Build history of the part. All positions in model axes, mm. A direction names the side the tool comes from. Coordinates: 2 decimals unless noted, no trailing zeros. Order: outer loops, then holes, each group sorted by start corner. A loop starts at its lowest first (then second) coordinate and runs counter-clockwise, first axis right, second up. Notation, with made-up numbers: M 27,80 L 77,80 A31 cw 77,111 Z; hole C 66.5,-18 d2. An arc over 180 degrees is marked long. Write item = value, one per line. Start each with the question number.
Q1. Pull direction X, two halves, no side cores. Call faces 1 (the face through (0, -7, 0)), 2 (the face through (18.417, -4.984, 14.383)), 3 (the face through (-3, -22, 20)): released by +X, released by -X, zero draft, split by the parting line, or undercut.
Q2. Band-saw the part on D-D on x = -4. Write the cut outline in (y, z), plus the area to 3 significant figures.
Q3. Drill centre lines: probe 1 along X at (y, z) = (-5.75, 6); probe 2 along X at (y, z) = (-13, 37.5); probe 3 along Y at (x, z) = (17, 22.5). Where is each one in solid material? Low to high.
Q4. Band-saw the part on C-C on y = -15. Write the cut outline in (x, z), plus the area to 3 significant figures.
Q5. Band-saw the part on A-A on x = -20. Write the cut outline in (y, z) (3 decimals), plus the area to 3 significant figures.
Q6. Pin check, flat tips, straight feed: P1, Ø5, axis at x = 1.5, y = -7.5, coming from the +Z side; P2, Ø7, axis at x = -20, z = 6, coming from the +Y side; P3, Ø4, axis at x = -12.5, z = 28.5, coming from the -Y side; P4, Ø17, axis at y = -5.34, z = 22.5, coming from the -X side. Stop position of each tip, or through.
Q7. Band-saw the part on B-B on z = 6. State how many separate pieces and enclosed holes the cut face has, plus the area to 3 significant figures.
Q8. 3-axis set-ups, long thin cutter, end or side, ignore diameter. For faces 4 (the face through (22.948, -5.055, 16.006)), 5 (the face through (24.46, 6.69, 5.41)), 6 (the face through (15.952, -12, 29)): which of +Z, -Z, +X, -X, +Y, -Y reach the whole face in a straight line?
```python
from build123d import *

# Parameters (mm, degrees)
BOSS_EXTRUDE1_DEPTH = 40
SKETCH2_R           = 2.6
BOSS_EXTRUDE2_DEPTH = 9
SKETCH3_R           = 4.5
CUT_EXTRUDE1_DEPTH  = 5
SKETCH4_R           = 2.6
CUT_EXTRUDE2_DEPTH  = 59.309518948
CHAMFER1_SIZE       = 3
SKETCH5_R           = 6.5
CUT_EXTRUDE3_DEPTH  = 55
SKETCH6_R           = 8.125
CUT_EXTRUDE4_DEPTH  = 5
CUT_EXTRUDE5_START  = -5
SKETCH7_R           = 8.125
CUT_EXTRUDE5_DEPTH  = 5
SKETCH8_R           = 8.125
CUT_EXTRUDE6_DEPTH  = 5
SKETCH9_R           = 4.5
CUT_EXTRUDE7_DEPTH  = 4
CHAMFER2_SIZE       = 3
SKETCH10_W          = 6
SKETCH10_H          = 40
BOSS_EXTRUDE3_DEPTH = 2
CUT_EXTRUDE8_DEPTH  = 5
CUT_EXTRUDE9_DEPTH  = 36


with BuildPart() as part:
    # Sketch1 → Boss-Extrude1 (new body)
    with BuildSketch(Plane.XY):
        Polygon((30, -21.341245707), (30, 8.658754293), (7.5, 8.658754293), (7.502146126, 4.017294787), (15.952208639, 4.017294787), (15.952208639, -17.982705213), (-15.952208639, -17.982705213), (-15.952208639, 4.017294787), (-7.502146126, 4.017294787), (-7.5, 8.658754293), (-30, 8.658754293), (-30, -21.341245707), align=None)
    extrude(amount=BOSS_EXTRUDE1_DEPTH)

    # Sketch2 → Boss-Extrude2 (add)
    with BuildSketch(Plane(origin=(0, 0, 0), x_dir=(-1, 0, 0), z_dir=(0, 0, -1))):
        Polygon((-7.502146126, -0.25363415), (-7.502146126, 4.017294787), (-15.952208639, 4.017294787), (-15.952208639, -17.982705213), (-5.499999997, -17.982705213), (-5.499999997, -13.845664874), (-4.999999997, -13.345655401), (5.020834238, -13.345465543), (5.518750814, -13.845451729), (5.50151136, -17.982705213), (15.952208639, -17.982705213), (15.952208639, 4.017294787), (7.502146126, 4.017294787), (7.504120794, -0.253349836), align=None)
        with Locations((-9.99998, -11.341245707)):
            Circle(SKETCH2_R, mode=Mode.SUBTRACT)
        with Locations((9.99998, -11.341245707)):
            Circle(SKETCH2_R, mode=Mode.SUBTRACT)
    extrude(amount=-BOSS_EXTRUDE2_DEPTH)

    # Sketch3 → Cut-Extrude1 (cut)
    with BuildSketch(Plane.XY.offset(9)):
        with Locations((-9.99998, -11.341245707)):
            Circle(SKETCH3_R)
        with Locations((9.99998, -11.341245707)):
            Circle(SKETCH3_R)
    extrude(amount=-CUT_EXTRUDE1_DEPTH, mode=Mode.SUBTRACT)

    # Sketch4 → Cut-Extrude2 (cut, through all)
    with BuildSketch(Plane(origin=(0, 8.658754293, 0), x_dir=(1, 0, 0), z_dir=(0, 1, 0))):
        with Locations(Location((-20, -6, 0), (0, 0, 270))):
            Circle(SKETCH4_R)
        with Locations(Location((20, -6, 0), (0, 0, 90))):
            Circle(SKETCH4_R)
    extrude(amount=-CUT_EXTRUDE2_DEPTH, mode=Mode.SUBTRACT)

    # Chamfer1
    # the kernel refuses this chamfer: 3 mm, written as the material it adds along each edge
    with BuildSketch(Plane(origin=(15.952208639, 4.017294787, 9), x_dir=(0.02749587661058678, 0, 0.9996219169112968), z_dir=(0, -1, 0))) as chamfer1_piece_1_section:
        Polygon((CHAMFER1_SIZE * 0.999621916911, CHAMFER1_SIZE * 0.0274958766106), (-CHAMFER1_SIZE * 0.0274958766106, CHAMFER1_SIZE * 0.999621916911), (0, 0), align=None)
    chamfer1_piece_1 = extrude(amount=22, mode=Mode.PRIVATE)
    chamfer1_piece_1 = chamfer1_piece_1 - Plane(origin=(9.99998, -11.341245707, 10.026917349), x_dir=(1, 0, 0), z_dir=(0, 0, 1)) * Cylinder(4.5, 56, mode=Mode.PRIVATE)
    add(chamfer1_piece_1)
    with BuildSketch(Plane(origin=(-15.952208639, -17.982705213, 9), x_dir=(-0.02749587661058678, 0, 0.9996219169112968), z_dir=(0, 1, 0))) as chamfer1_piece_2_section:
        Polygon((CHAMFER1_SIZE * 0.999621916911, CHAMFER1_SIZE * 0.0274958766106), (-CHAMFER1_SIZE * 0.0274958766106, CHAMFER1_SIZE * 0.999621916911), (0, 0), align=None)
    chamfer1_piece_2 = extrude(amount=22, mode=Mode.PRIVATE)
    chamfer1_piece_2 = chamfer1_piece_2 - Plane(origin=(-9.99998, -11.341245707, 10.026917349), x_dir=(1, 0, 0), z_dir=(0, 0, 1)) * Cylinder(4.5, 56, mode=Mode.PRIVATE)
    add(chamfer1_piece_2)

    # Sketch5 → Cut-Extrude3 (cut)
    with BuildSketch(Plane.ZY.offset(30)):
        with Locations((22.5, -5.341245707)):
            Circle(SKETCH5_R)
    extrude(amount=-CUT_EXTRUDE3_DEPTH, mode=Mode.SUBTRACT)

    # Sketch6 → Cut-Extrude4 (cut)
    with BuildSketch(Plane.ZY.offset(30)):
        with Locations((22.5, -5.341245707)):
            Circle(SKETCH6_R)
    extrude(amount=-CUT_EXTRUDE4_DEPTH, mode=Mode.SUBTRACT)

    # Sketch7 → Cut-Extrude5 (cut)
    with BuildSketch(Plane(origin=(-15.952208639, 0, 0), x_dir=(0, 0, -1), z_dir=(1, 0, 0)).offset(CUT_EXTRUDE5_START)):
        with Locations(Location((-22.5, -5.341245707, 0), (0, 0, 180))):
            Circle(SKETCH7_R)
    extrude(amount=CUT_EXTRUDE5_DEPTH, mode=Mode.SUBTRACT)

    # Sketch8 → Cut-Extrude6 (cut)
    with BuildSketch(Plane.ZY.offset(-15.952208639)):
        with Locations((22.5, -5.341245707)):
            Circle(SKETCH8_R)
    extrude(amount=-CUT_EXTRUDE6_DEPTH, mode=Mode.SUBTRACT)

    # Sketch9 → Cut-Extrude7 (cut)
    with BuildSketch(Plane(origin=(0, 8.658754293, 0), x_dir=(1, 0, 0), z_dir=(0, 1, 0))):
        with Locations(Location((20, -6, 0), (0, 0, 270))):
            Circle(SKETCH9_R)
        with Locations(Location((-20, -6, 0), (0, 0, 270))):
            Circle(SKETCH9_R)
    extrude(amount=-CUT_EXTRUDE7_DEPTH, mode=Mode.SUBTRACT)

    # Chamfer2
    chamfer2_edges = [part.edges().sort_by_distance(p)[0] for p in [
        (30, 8.658754293, 20),
        (-30, 8.658754293, 20),
    ]]
    chamfer(chamfer2_edges, length=CHAMFER2_SIZE)

    # Sketch10 → Boss-Extrude3 (add)
    with BuildSketch(Plane.XZ.offset(21.341245707)):
        with Locations((0, 20)):
            Rectangle(SKETCH10_W, SKETCH10_H)
    extrude(amount=BOSS_EXTRUDE3_DEPTH)

    # Sketch11 → Cut-Extrude8 (cut)
    with BuildSketch(Plane.XY.offset(9)):
        with BuildLine():
            Line((9.99998, -6.841245707), (-9.99998, -6.841245707))
            ThreePointArc((-9.99998, -6.841245707), (-5.784946566, -12.917155968), (-12.952208639, -14.737470974))
            Line((-12.952208639, -14.737470974), (-12.952208639, -17.982705213))
            Line((-12.952208639, -17.982705213), (-5.50151136, -17.982705213))
            Line((-5.50151136, -17.982705213), (-5.518750814, -13.845451729))
            Line((-5.518750814, -13.845451729), (-5.020834238, -13.345465543))
            Line((-5.020834238, -13.345465543), (4.999999997, -13.345655401))
            Line((4.999999997, -13.345655401), (5.499999997, -13.845664874))
            Line((5.499999997, -13.845664874), (5.499999997, -17.982705213))
            Line((5.499999997, -17.982705213), (12.952208639, -17.982705213))
            Line((12.952208639, -17.982705213), (12.952208639, -14.737470974))
            ThreePointArc((12.952208639, -14.737470974), (5.784946566, -12.917155968), (9.99998, -6.841245707))
        make_face()
        with BuildLine():
            Line((-12.952208639, -17.982705213), (-12.952208639, -14.737470974))
            ThreePointArc((-12.952208639, -14.737470974), (-14.081267005, -13.236792167), (-14.499514384, -11.405978467))
            Line((-14.499514384, -11.405978467), (-14.452208639, -17.982705213))
            Line((-14.452208639, -17.982705213), (-12.952208639, -17.982705213))
        make_face()
        with BuildLine():
            ThreePointArc((14.499514384, -11.405978467), (14.081267005, -13.236792167), (12.952208639, -14.737470974))
            Line((12.952208639, -14.737470974), (12.952208639, -17.982705213))
            Line((12.952208639, -17.982705213), (14.452208639, -17.982705213))
            Line((14.452208639, -17.982705213), (14.499514384, -11.405978467))
        make_face()
    extrude(amount=-CUT_EXTRUDE8_DEPTH, mode=Mode.SUBTRACT)

    # Sketch13 → Cut-Extrude9 (cut)
    with BuildSketch(Plane.XY.offset(40)):
        Polygon((-14.49998, -11.341245707), (-14.452208639, -17.982705213), (14.452208639, -17.982705213), (14.49998, -11.341245707), align=None)
    extrude(amount=-CUT_EXTRUDE9_DEPTH, mode=Mode.SUBTRACT)


solid = part.part
```
Recorded:
q1.face_1 = zero draft
q1.face_2 = undercut
q1.face_3 = released by -X
q2.outline = M -21.34,0 L -17.98,0 L -17.98,40 L -21.34,40 Z; M -13.35,0 L -0.25,0 L -0.25,9 L -6.84,9 L -6.84,4 L -13.35,4 Z
q2.area = 220 mm2
q3.probe_1 = -30 to -22.6, -17.4 to 17.4, 22.6 to 30
q3.probe_2 = -30 to -15.95, 15.95 to 30
q3.probe_3 = -21.34 to -13.47, 2.78 to 8.66
q4.outline = M -30,0 L -5.51,0 L -5.51,4 L -14.47,4 L -14.47,10.52 L -15.95,12 L -15.95,40 L -30,40 Z; M 5.5,0 L 30,0 L 30,40 L 15.95,40 L 15.95,12 L 14.47,10.52 L 14.47,4 L 5.5,4 Z; hole C -20,6 d5.2; hole C 20,6 d5.2
q4.area = 1,190 mm2
q5.outline = M -21.341,0 L 8.659,0 L 8.659,1.5 L 4.659,1.5 L 4.659,3.4 L -21.341,3.4 Z; M -21.341,8.6 L 4.659,8.6 L 4.659,10.5 L 8.659,10.5 L 8.659,40 L -21.341,40 Z; hole C -5.341,22.5 d16.25
q5.area = 821 mm2
q6.P1 = 9
q6.P2 = 4.66
q6.P3 = -21.34
q6.P4 = -30
q7.separate_pieces = 3
q7.enclosed_holes = 1
q7.area = 1,010 mm2
q8.face_4 = -X
q8.face_5 = +Y
q8.face_6 = +Z
